```python
from build123d import *

# Parameters (mm, degrees)
PAD_DEPTH    = 1
SKETCH001_R  = 5.16
SKETCH001_W  = 33.87
SKETCH001_H  = 11.9
PAD001_DEPTH = 1
FILLET_R     = 1


with BuildPart() as part:
    # Sketch → Pad (new body)
    with BuildSketch(Plane.XY):
        with BuildLine():
            Line((2, 54), (122, 54))
            ThreePointArc((124, 52), (123.414214, 53.414214), (122, 54))
            Line((124, 52), (124, 2))
            ThreePointArc((122, 0), (123.414214, 0.585786), (124, 2))
            Line((122, 0), (2, 0))
            ThreePointArc((0, 2), (0.585786, 0.585786), (2, 0))
            Line((0, 2), (0, 52))
            ThreePointArc((2, 54), (0.585786, 53.414214), (0, 52))
        make_face()
    extrude(amount=PAD_DEPTH)

    # Sketch001 (on Face10 of Pad) → Pad001 (join)
    with BuildSketch(Plane.XY.offset(1)):
        with BuildLine():
            ThreePointArc((2, 54), (0.585786, 53.414214), (0, 52))
            Line((0, 2), (0, 52))
            ThreePointArc((0, 2), (0.585786, 0.585786), (2, 0))
            Line((122, 0), (2, 0))
            ThreePointArc((122, 0), (123.414214, 0.585786), (124, 2))
            Line((124, 52), (124, 2))
            ThreePointArc((124, 52), (123.414214, 53.414214), (122, 54))
            Line((2, 54), (122, 54))
        make_face()
        with BuildLine():
            Line((4, 52), (120, 52))
            ThreePointArc((122, 50), (121.414214, 51.414214), (120, 52))
            Line((122, 50), (122, 4))
            ThreePointArc((120, 2), (121.414214, 2.585786), (122, 4))
            Line((120, 2), (4, 2))
            ThreePointArc((2, 4), (2.585786, 2.585786), (4, 2))
            Line((2, 4), (2, 50))
            ThreePointArc((4, 52), (2.585786, 51.414214), (2, 50))
        make_face(mode=Mode.SUBTRACT)
        with Locations((87.175, 15.665)):
            Circle(SKETCH001_R)
        with Locations((103.335, 15.665)):
            Circle(SKETCH001_R)
        Polygon((9.48, 26.12), (16.5, 26.12), (16.5, 33.14), (26.8, 33.14), (26.8, 26.12), (33.82, 26.12), (33.82, 15.82), (26.8, 15.82), (26.8, 8.8), (16.5, 8.8), (16.5, 15.82), (9.48, 15.82), align=None)
        with Locations((57.075, 15.665)):
            Rectangle(SKETCH001_W, SKETCH001_H)
    extrude(amount=PAD001_DEPTH)

    # Fillet
    fillet_edges = [part.edges().sort_by_distance(p)[0] for p in [
        (26.8, 15.82, 1.5),
        (33.82, 15.82, 1.5),
        (33.82, 26.12, 1.5),
        (26.8, 33.14, 1.5),
        (74.01, 9.715, 1.5),
        (74.01, 21.615, 1.5),
        (40.14, 9.715, 1.5),
        (26.8, 8.8, 1.5),
        (16.5, 8.8, 1.5),
        (9.48, 15.82, 1.5),
        (26.8, 26.12, 1.5),
        (40.14, 21.615, 1.5),
        (16.5, 33.14, 1.5),
        (9.48, 26.12, 1.5),
        (16.5, 26.12, 1.5),
        (16.5, 15.82, 1.5),
    ]]
    fillet(fillet_edges, radius=FILLET_R)


solid = part.part
```
The listing builds one solid part. Answer for the finished solid, in the listing's coordinates (mm). A direction names the side the tool comes from. Give positions to 0.01 mm unless a question says otherwise; leave off trailing zeros. Loops run counter-clockwise (first coordinate to the right, second up) from the corner with the lowest first, then second, coordinate; pieces in that order, holes last. Notation, with made-up numbers: M -33.5,-23 L 7.5,-23 A4 cw 7.5,-18 Z; hole C 72.5,87 d8. An arc over 180 degrees is marked long. One line per item, written item: value.
1. Find the intervals of material crossed by probe 1 along Y at (x, z) = (69, 1.65) (3 decimals); probe 2 along Y at (x, z) = (108, 1.05); probe 3 along X at (y, z) = (49.5, 1.8), in increasing order.
Found:
probe 1: 0 to 2, 9.715 to 21.615, 52 to 54
probe 2: 0 to 2, 13.46 to 17.87, 52 to 54
probe 3: 0 to 2, 122 to 124
2. Section D-D on x = 64 is taken. Determine the outline of the cut face in (y, z) (3 decimals), plus the area to 3 significant figures.
Found:
outline: M 0,0 L 54,0 L 54,2 L 52,2 L 52,1 L 21.615,1 L 21.615,2 L 9.715,2 L 9.715,1 L 2,1 L 2,2 L 0,2 Z
area: 69.9 mm^2
3. For a pull along X with two mould halves and no side action, classify faces 3 (the face through (87, 16, 2)), 4 (the face through (63, 27, 1)) as pulls with the +X half, pulls with the -X half, needs draft (parallel to the pull), parting line crosses it, or undercut.
Found:
face 3: needs draft
face 4: undercut
4. Section C-C on z = 1.3 is taken. State how many separate pieces and enclosed holes the cut face has, plus the area to 3 significant figures.
Found:
separate pieces: 5
enclosed holes: 1
area: 1,660 mm^2
5. For faces 1 (the face through (63, 27, 0)), 2 (the face through (92.1, 17.2, 1.5)), determine the directions among +Z, -Z, +X, -X, +Y, -Y from which every point of the face is accessible in a straight line to the end or side of a thin tool.
Found:
face 1: -Z, +X, -X, +Y, -Y
face 2: +Z
6. Section A-A on x = 79.5 is taken. Determine the outline of the cut face in (y, z).
Found:
outline: M 0,0 L 54,0 L 54,2 L 52,2 L 52,1 L 2,1 L 2,2 L 0,2 Z
7. Section B-B on y = 36 is taken. Determine the outline of the cut face in (x, z), plus the area to 3 significant figures.
Found:
outline: M 0,0 L 124,0 L 124,2 L 122,2 L 122,1 L 2,1 L 2,2 L 0,2 Z
area: 128 mm^2
